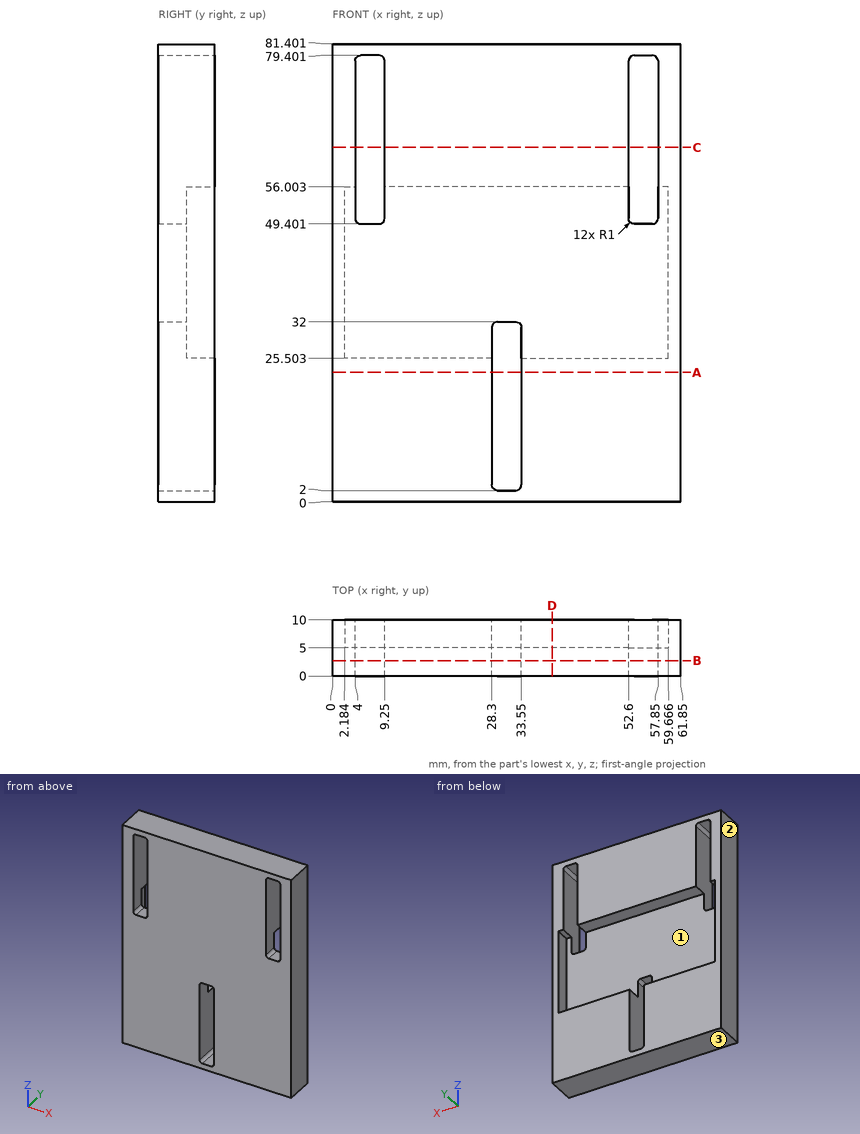
Print and shaded views of the part. All mm, measured from the part's lowest x, y and z. Give positions to 0.01 mm unless a question says otherwise; leave off trailing zeros. Loops run counter-clockwise (first coordinate to the right, second up) from the corner with the lowest first, then second, coordinate; pieces in that order, holes last. Notation, with made-up numbers: (19, 75) - (52, 75) arc R22 cw to (52, 92) - close; hole circle Ø1 at (78.25, 73.5). An arc over 180 degrees is marked (long way). One line per item, written item: value. Start each with the question number.
1. Slice it at D-D (x = 39). List the corners of the cut face in (y, z).
2. Pin check, flat tip, straight feed: pin 1 (2.5 mm diameter, centred on x = 55, y = 3, fed in from -Z). Stop position of the tip, or through.
3. Slice it at A-A (z = 23). List the corners of the cut face in (x, y), plus the area to 3 significant figures.
4. Probe L1, parallel to X at y = 9.75, z = 76; L2, parallel to X at y = 2, z = 26; L3, parallel to Z at x = 27.5, y = 5.75. List the from-to ranges inside material, lowest first. Write a range as from..to.
5. Pull direction Z, two halves, no side cores. Call the marked faces 1, 2 and 3: pulls with the +Z half, pulls with the -Z half, needs draft (parallel to the pull), parting line crosses it, or undercut.
6. Slice it at B-B (y = 2.75). List the corners of the cut face in (x, z).
7. Slice it at C-C (z = 63). List the corners of the cut face in (x, y).
Solution:
1. outline: (0, 0) - (10, 0) - (10, 25.5) - (5, 25.5) - (5, 56) - (10, 56) - (10, 81.4) - (0, 81.4) - close
2. pin 1: stops at z = 0
3. outline: (0, 0) - (28.3, 0) - (28.3, 10) - (0, 10) - close; (33.55, 0) - (61.85, 0) - (61.85, 10) - (33.55, 10) - close
3. area: 566 mm^2
4. L1: x = 0..4, 9.25..52.6, 57.85..61.85
4. L2: x = 0..28.3, 33.55..61.85
4. L3: z = 0..25.5, 56..81.4
5. face 1: undercut
5. face 2: needs draft
5. face 3: pulls with the -Z half
6. outline: (0, 0) - (61.85, 0) - (61.85, 81.4) - (0, 81.4) - close; hole (4, 50.4) arc R1 ccw to (5, 49.4) - (8.25, 49.4) arc R1 ccw to (9.25, 50.4) - (9.25, 78.4) arc R1 ccw to (8.25, 79.4) - (5, 79.4) arc R1 ccw to (4, 78.4) - close; hole (28.3, 3) arc R1 ccw to (29.3, 2) - (32.55, 2) arc R1 ccw to (33.55, 3) - (33.55, 31) arc R1 ccw to (32.55, 32) - (29.3, 32) arc R1 ccw to (28.3, 31) - close; hole (52.6, 50.4) arc R1 ccw to (53.6, 49.4) - (56.85, 49.4) arc R1 ccw to (57.85, 50.4) - (57.85, 78.4) arc R1 ccw to (56.85, 79.4) - (53.6, 79.4) arc R1 ccw to (52.6, 78.4) - close
7. outline: (0, 0) - (4, 0) - (4, 10) - (0, 10) - close; (9.25, 0) - (52.6, 0) - (52.6, 10) - (9.25, 10) - close; (57.85, 0) - (61.85, 0) - (61.85, 10) - (57.85, 10) - close
